Autodesk Inventor part; units mm, degrees
ref_plane "YZ Plane" through (0, 0, 0) normal (1, 0, 0) x (0, 1, 0)
ref_plane "XZ Plane" through (0, 0, 0) normal (0, 1, 0) x (-1, 0, 0)
ref_plane "XY Plane" through (0, 0, 0) normal (0, 0, 1) x (1, 0, 0)
sketch "Sketch1" plane through (0, 0, 0) normal (0, 0, 1) x (1, 0, 0)
  line L0 (-75, 60) -> (75, 60)
  line L1 (75, 60) -> (75, -60)
  line L2 (75, -60) -> (-75, -60)
  line L3 (-75, -60) -> (-75, 60)
  point P0 (0, 0)
  dimension "d0" = 150
  dimension "d1" = 120
  dimension "d2" = 60
  dimension "d3" = 75
extrude "Extrusion1" add sketch "Sketch1" along normal blind 6.35
sketch "Sketch2" plane through (0, 0, 6.35) normal (0, 0, 1) x (1, 0, 0)
  line L0 (-75, 60) -> (-75, -60)
  line L1 (-75, 40) -> (-68.65, 40)
  line L2 (-68.65, 40) -> (-68.65, 20)
  line L3 (-68.65, 20) -> (-75, 20)
  line L4 (-75, 20) -> (-75, 40)
  line L5 (-75, 60) -> (-75, -60)
  line L6 (-75, 0) -> (-68.65, 0)
  line L7 (-68.65, 0) -> (-68.65, -20)
  line L8 (-68.65, -20) -> (-75, -20)
  line L9 (-75, -20) -> (-75, 0)
  line L10 (-75, -40) -> (-68.65, -40)
  line L11 (-68.65, -40) -> (-68.65, -60)
  line L12 (-68.65, -60) -> (-75, -60)
  line L13 (-75, -60) -> (-75, -40)
  line L14 (75, -60) -> (75, 60)
  line L15 (75, 40) -> (68.65, 40)
  line L16 (68.65, 40) -> (68.65, 20)
  line L17 (68.65, 20) -> (75, 20)
  line L18 (75, 20) -> (75, 40)
  line L19 (75, 0) -> (68.65, 0)
  line L20 (68.65, 0) -> (68.65, -20)
  line L21 (68.65, -20) -> (75, -20)
  line L22 (75, -20) -> (75, 0)
  line L23 (75, -40) -> (68.65, -40)
  line L24 (68.65, -40) -> (68.65, -60)
  line L25 (68.65, -60) -> (75, -60)
  line L26 (75, -60) -> (75, -40)
  line L27 (-75, -60) -> (75, -60)
  line L28 (-28.65, -60) -> (28.65, -60)
  line L29 (28.65, -60) -> (28.65, -53.65)
  line L30 (28.65, -53.65) -> (-28.65, -53.65)
  line L31 (-28.65, -53.65) -> (-28.65, -60)
  line L32 (75, 60) -> (-75, 60)
  line L33 (-28.65, 60) -> (28.65, 60)
  point P0 (0, 0)
  dimension "d6" = 6.35
  dimension "d7" = 20
  dimension "d8" = 20
  dimension "d9" = 20
  dimension "d10" = 20
  dimension "d11" = 20
  dimension "d12" = 20
  dimension "d13" = 20
  dimension "d22" = 57.3
  dimension "d23" = 46.35
  dimension "d24" = 46.35
  dimension "d26" = 6.35
extrude "Extrusion2" cut sketch "Sketch2" against normal through all contours L1 L2 L3 L0 | L6 L7 L8 L0 | L14 L17 L16 L15 | L10 L11 L12 L0 | L14 L21 L20 L19 | L31 L30 L29 L27 | L14 L25 L24 L23
sketch "Sketch3" plane through (0, 0, 6.35) normal (0, 0, 1) x (1, 0, 0)
  circle A0 centre (0, -4.5) radius 27
  line L0 (-75, -60) -> (75, -60)
  line L1 (75, 40) -> (75, 60)
  point P0 (0, 0)
  dimension "d16" = 55.5
  dimension "d17" = 75
  dimension "d18" = 54
extrude "Extrusion3" cut sketch "Sketch3" against normal through all
sketch "Sketch4" plane through (0, 0, 6.35) normal (0, 0, 1) x (1, 0, 0)
  circle A0 centre (0, -4.5) radius 27
  circle A1 centre (0, -4.5) radius 33.5
  circle A2 centre (23.6881, 19.1881) radius 1.75
  line L0 (0, -4.5) -> (33.5, -4.5)
  line L1 (0, -4.5) -> (23.6881, 19.1881)
  point P0 (0, 0)
  dimension "d27" = 67
  dimension "d28" = 45
  dimension "d29" = 3.5
extrude "Extrusion4" cut sketch "Sketch4" against normal through all contours L1 A1 A2 | A2 A1 L1 | A1 A2
pattern_circular "Circular Pattern1" count 4 over 360 about axis through (0, -4.5, 6.35) along (0, 0, -1) of "Extrusion4"
sketch "Sketch5" plane through (0, 0, 6.35) normal (0, 0, 1) x (1, 0, 0)
  circle A0 centre (-54.9, -48) radius 1.75
  circle A1 centre (54.9, -48) radius 1.75
  line L0 (-68.65, -60) -> (-28.65, -60)
  line L1 (-75, -20) -> (-75, -40)
  line L2 (75, -40) -> (75, -20)
  line L3 (28.65, -60) -> (68.65, -60)
  point P0 (0, 0)
  dimension "d35" = 3.5
  dimension "d36" = 12
  dimension "d37" = 20.1
  dimension "d38" = 20.1
  dimension "d39" = 12
extrude "Extrusion5" cut sketch "Sketch5" against normal blind 10
equation "\"d11\" = d8"
equation "\"d12\" = d9"
equation "\"d13\" = d10"
equation "\"d22\" = d21"
equation "\"d24\" = d23"
equation "\"d26\" = d25"
properties part number "2204_Housing Front_V1" material "Wood (Birch)"
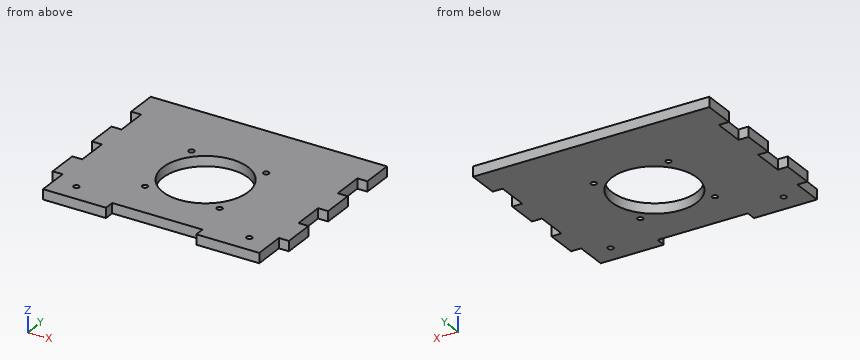
Read the model definition and answer for the solid it produces. Units are mm, in the model's axes. Coordinates: 2 decimals unless noted, no trailing zeros. Order: outer loops, then holes, each group sorted by start corner. A loop starts at its lowest first (then second) coordinate and runs counter-clockwise, first axis right, second up. Notation, with made-up numbers: (-27, 89.5) - (10, 89.5) arc R7 cw to (10, 101.5) - close; hole circle Ø8 at (73.5, -9.75). An arc over 180 degrees is marked (long way). Answer as a JSON object with one key per item and string values. Group by question number.
Item 1: Consider probe 1 along Y at (x, z) = (54.9, 2.5); probe 2 along X at (y, z) = (-55, 5); probe 3 along Y at (x, z) = (-23.5, 1.75). Determine where each line is inside the solid, lowest interval first. Write a range as from..to.
Item 2: Section A-A (x = 54.9) is taken. Give the vertices of the cut face in (y, z), plus the area to 3 significant figures.
Item 3: Section D-D (z = 1.25) is taken. State how many separate pieces and enclosed holes the cut face has, plus the area to 3 significant figures.
Item 4: Section B-B (y = -4.5) is taken. Give the vertices of the cut face in (x, z), plus the area to 3 significant figures.
Item 5: Flat-ended cylindrical pins translate along their axes: P1, Ø5.5, axis at x = -23.69, y = 19.19, coming from the +Z side; P2, Ø3, axis at x = -71, z = 4, coming from the -Y side; P3, Ø2, axis at y = -45.5, z = 5.5, coming from the -X side; P4, Ø3, axis at x = 11.5, z = 3, coming from the -Y side. Find the tip coordinate at first contact, or state that the pin passes through.
Item 6: Section C-C (y = -42.5) is taken. Give the vertices of the cut face in (x, z), plus the area to 3 significant figures.
Results are:
{
 "1": {"probe 1": "y = -60..-49.75, -46.25..60", "probe 2": "x = -68.65..-28.65, 28.65..68.65", "probe 3": "y = -53.65..-29.93, -26.45..-17.79, 8.79..17.45, 20.93..60"},
 "2": {"outline": "(-60, 0) - (-49.75, 0) - (-49.75, 6.35) - (-60, 6.35) - close; (-46.25, 0) - (60, 0) - (60, 6.35) - (-46.25, 6.35) - close", "area": "740 mm^2"},
 "3": {"separate pieces": "1", "enclosed holes": "7", "area": "14,500 mm^2"},
 "4": {"outline": "(-68.65, 0) - (-27, 0) - (-27, 6.35) - (-68.65, 6.35) - close; (27, 0) - (68.65, 0) - (68.65, 6.35) - (27, 6.35) - close", "area": "529 mm^2"},
 "5": {"P1": "stops at z = 6.35", "P2": "stops at y = -40", "P3": "stops at x = -68.65", "P4": "stops at y = -53.65"},
 "6": {"outline": "(-68.65, 0) - (68.65, 0) - (68.65, 6.35) - (-68.65, 6.35) - close", "area": "872 mm^2"}
}
